Check sheet for the modelled part. Datum: model origin and axes. Units: mm. Face numbers are marked on the shaded views. Round coordinates to 2 decimals unless told otherwise and drop trailing zeros. Loops run counter-clockwise (first coordinate to the right, second up) from the corner with the lowest first, then second, coordinate; pieces in that order, holes last. Notation, with made-up numbers: (34.25, 36) -> (90.25, 36) arc R27 ccw to (90.25, 58) -> close; hole circle Ø1 at (79.5, -27.75). An arc over 180 degrees is marked (long way). Return JSON: item names as keys, results as strings.
from build123d import *

# Parameters (mm, degrees)
EXTRUDE_1_DEPTH          = 140
CUT_EXTRUDE_1_DEPTH      = 20
CUT_EXTRUDE_1_DEPTH_BACK = 20
SKETCH_2_W               = 78.4
SKETCH_2_H               = 11
CUT_EXTRUDE_2_DEPTH      = 78.4
CUT_EXTRUDE_2_DEPTH_BACK = 207.820308481
SKETCH_3_R               = 3.2
FILLET_1_R               = 1
SKETCH_4_W               = 14.133249581
SKETCH_4_H               = 78.4
CUT_EXTRUDE_3_DEPTH      = 225.379143416
CUT_EXTRUDE_4_DEPTH      = 225.379143416
CUT_EXTRUDE_4_DEPTH_BACK = 225.379143416
SKETCH_5_W               = 136.544306781
SKETCH_5_H               = 100


with BuildPart() as part:
    # 草图1 → 凸台-拉伸1 (new body)
    with BuildSketch(Plane.XY):
        with BuildLine():
            Line((0, 0), (175, 0))
            Line((175, 0), (175, 4))
            Line((175, 4), (167.055676963, 10))
            Line((167.055676963, 10), (167.055676963, 4))
            Line((167.055676963, 4), (164.053399387, 4))
            Line((164.053399387, 4), (156.10907635, 10))
            Line((156.10907635, 10), (156.10907635, 4))
            Line((156.10907635, 4), (153.106798774, 4))
            Line((153.106798774, 4), (145.162475737, 10))
            Line((145.162475737, 10), (145.162475737, 4))
            Line((145.162475737, 4), (142.160198161, 4))
            Line((142.160198161, 4), (134.215875124, 10))
            Line((134.215875124, 10), (134.215875124, 4))
            Line((134.215875124, 4), (131.213597548, 4))
            Line((131.213597548, 4), (123.269274511, 10))
            Line((123.269274511, 10), (123.269274511, 4))
            Line((123.269274511, 4), (120.266996935, 4))
            Line((120.266996935, 4), (112.322673898, 10))
            Line((112.322673898, 10), (112.322673898, 4))
            Line((112.322673898, 4), (109.320396322, 4))
            Line((109.320396322, 4), (101.376073285, 10))
            Line((101.376073285, 10), (101.376073285, 4))
            Line((101.376073285, 4), (98.373795709, 4))
            Line((98.373795709, 4), (90.429472672, 10))
            Line((90.429472672, 10), (90.429472672, 4))
            Line((90.429472672, 4), (72.427195096, 4))
            Line((72.427195096, 4), (65.557646205, 4))
            Line((65.557646205, 4), (61.480594483, 4))
            Line((61.480594483, 4), (54.611045592, 4))
            Line((54.611045592, 4), (6.633249581, 4))
            ThreePointArc((6.633249581, 4), (-3.872983346, 13.922616289), (0, 0))
        make_face()
        Polygon((3.2, 7.5), (1.6, 10.271281292), (-1.6, 10.271281292), (-3.2, 7.5), (-1.6, 4.728718708), (1.6, 4.728718708), align=None, mode=Mode.SUBTRACT)
    extrude(amount=-EXTRUDE_1_DEPTH)

    # 草图2 → 切除-拉伸1 (cut, two sides: drawn at the far end of the back side and taken through both)
    with BuildSketch(Plane(origin=(0, 0, 0), x_dir=(0, 0, -1), z_dir=(1, 0, 0)).offset(-CUT_EXTRUDE_1_DEPTH_BACK)):
        with Locations((70, 9.5)):
            Rectangle(SKETCH_2_W, SKETCH_2_H)
    extrude(amount=CUT_EXTRUDE_1_DEPTH + CUT_EXTRUDE_1_DEPTH_BACK, mode=Mode.SUBTRACT)

    # 草图3 → 切除-拉伸2 (cut, two sides: drawn at the far end of the back side and taken through both)
    with BuildSketch(Plane.XY.offset(-109.2).offset(-CUT_EXTRUDE_2_DEPTH_BACK)):
        with Locations((0, 7.5)):
            Circle(SKETCH_3_R)
    extrude(amount=CUT_EXTRUDE_2_DEPTH + CUT_EXTRUDE_2_DEPTH_BACK, mode=Mode.SUBTRACT)

    # 圆角1
    fillet_1_edges = [part.edges().sort_by_distance(p)[0] for p in [
        (175, 2, -140),
        (175, 2, 0),
        (90.429472672, 10, -70),
        (101.376073285, 10, -70),
        (112.322673898, 10, -70),
        (123.269274511, 10, -70),
        (134.215875124, 10, -70),
        (145.162475737, 10, -70),
        (156.10907635, 10, -70),
        (167.055676963, 10, -70),
        (175, 4, -70),
        (175, 0, -70),
    ]]
    fillet(fillet_1_edges, radius=FILLET_1_R)

    # 草图4 → 切除-拉伸3 (cut, through all)
    with BuildSketch(Plane(origin=(0, 4, 0), x_dir=(1, 0, 0), z_dir=(0, 1, 0))):
        with Locations((0.43337521, 70)):
            Rectangle(SKETCH_4_W, SKETCH_4_H)
    extrude(amount=-CUT_EXTRUDE_3_DEPTH, mode=Mode.SUBTRACT)

    # 草图5 → 切除-拉伸4 (cut, two sides: drawn at the far end of the back side and taken through both)
    with BuildSketch(Plane(origin=(0, 4, 0), x_dir=(1, 0, 0), z_dir=(0, 1, 0)).offset(-CUT_EXTRUDE_4_DEPTH_BACK)):
        with Locations((95.772153391, 70)):
            Rectangle(SKETCH_5_W, SKETCH_5_H)
    extrude(amount=CUT_EXTRUDE_4_DEPTH + CUT_EXTRUDE_4_DEPTH_BACK, mode=Mode.SUBTRACT)


solid = part.part
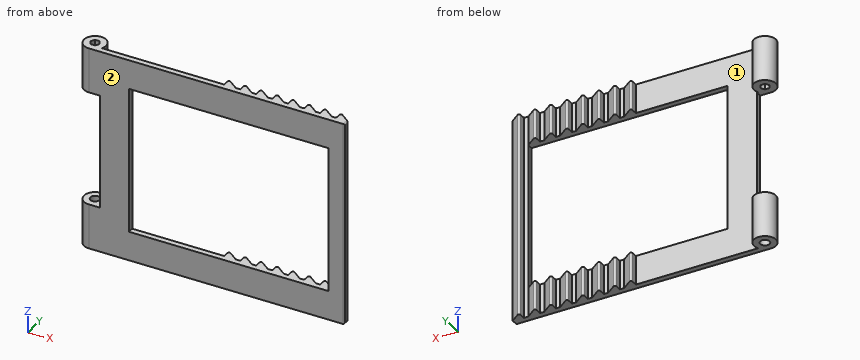
Q1. Section check D-D (x = 117). Record the boundary of the cut face in (y, z).
Results list:
{"outline": "(0, -140) -> (6.47, -140) -> (6.47, -120) -> (0, -120) -> close; (0, -20) -> (6.47, -20) -> (6.47, 0) -> (0, 0) -> close"}
Q2. Go/stop test with flat-tipped pins: pin 1 (4.5 mm diameter, centred on y = 6.5, z = -131, fed in from -X); pin 2 (1.5 mm diameter, centred on y = 10.5, z = -49.5, fed in from +X); pin 3 (3 mm diameter, centred on y = 3, z = -73, fed in from -X); pin 4 (2.5 mm diameter, centred on x = 143.5, z = -14, fed in from +Y). Record where each tip stops, or that it passes through.
Results list:
{"pin 1": "x = -7.5", "pin 2": "through", "pin 3": "x = 7.5", "pin 4": "y = 4"}
Q3. Material ranges on line 1 (Z direction, x = 103, y = 3.75); line 2 (Y direction, x = 0, z = -123); line 3 (Z direction, x = 5.5, y = 7), recorded low to high.
Results list:
{"line 1": "-140 to -120, -20 to 0", "line 2": "0 to 4.3, 10.7 to 15", "line 3": "-140 to -109.2, -30.8 to 0"}
Q4. Section check C-C (z = -26.5). Count the separate pieces of the cut face and the enclosed holes in it, then the cut area to 3 significant figures.
Results list:
{"separate pieces": "2", "enclosed holes": "1", "area": "308 mm^2"}
Q5. Section check B-B (x = 65.5). Record the boundary of the cut face in (y, z), then the cut area to 3 significant figures.
Results list:
{"outline": "(0, -140) -> (4, -140) -> (4, -120) -> (0, -120) -> close; (0, -20) -> (4, -20) -> (4, 0) -> (0, 0) -> close", "area": "160 mm^2"}
Q6. Draft check along X on the marked faces 1 and 2. Enter one of: released by +X, released by -X, zero draft, split by the parting line, or undercut.
Results list:
{"face 1": "undercut", "face 2": "zero draft"}
